```python
from build123d import *

# Parameters (mm, degrees)
F0_R           = 50.8
F1_DEPTH       = 38.1
F3_D           = 6.35
F4_D           = 12.7
F5_D           = 9.525
F5_CBORE_D     = 19.05
F5_CBORE_DEPTH = 6.35
F6_D           = 9.525
F6_CSINK_D     = 19.05
F6_CSINK_ANGLE = 82
F7_D           = 6.35


with BuildPart() as f1:
    # F0 (on Front) → F1 (new body)
    with BuildSketch(Plane.XZ):
        Circle(F0_R)
    extrude(amount=F1_DEPTH)

    # F3 (through all)
    with Locations(Plane(origin=(0, 0, 0), x_dir=(1, 0, 0), z_dir=(0, 1, 0))):
        with Locations((0, -31.75)):
            Hole(F3_D / 2)

    # F4 (through all)
    with Locations(Plane(origin=(0, 0, 0), x_dir=(1, 0, 0), z_dir=(0, 1, 0))):
        with Locations((-28.8894439592, -13.1705173676)):
            Hole(F4_D / 2)

    # F5 (through all)
    with Locations(Plane(origin=(0, 0, 0), x_dir=(1, 0, 0), z_dir=(0, 1, 0))):
        with Locations((28.8894439592, -13.1705173676)):
            CounterBoreHole(F5_D / 2, F5_CBORE_D / 2, F5_CBORE_DEPTH)

    # F6 (through all)
    with Locations(Plane(origin=(0, 0, 0), x_dir=(1, 0, 0), z_dir=(0, 1, 0))):
        with Locations((21.623259188, 23.2485948412)):
            CounterSinkHole(F6_D / 2, F6_CSINK_D / 2, counter_sink_angle=F6_CSINK_ANGLE)

    # F7 (through all)
    with Locations(Plane(origin=(0, 0, 0), x_dir=(1, 0, 0), z_dir=(0, 1, 0))):
        with Locations((-21.623259188, 23.2485948412)):
            Hole(F7_D / 2)


solid = f1.part
```
Geometry check sheet. Reference: the model listing, model coordinates, mm. A direction names the side the tool comes from. Give positions to 0.01 mm unless a question says otherwise; leave off trailing zeros. Order: outer loops, then holes, each group sorted by start corner. A loop starts at its lowest first (then second) coordinate and runs counter-clockwise, first axis right, second up. Notation, with made-up numbers: (-27.5, 75.25) - (24.5, 75.25) arc R30 cw to (24.5, 103.25) - close; hole circle Ø10 at (5.25, -25). An arc over 180 degrees is marked (long way). Answer in a Markdown table with one row per item. Add a question column.
Q1. Cross-section at C-C, the plane y = -13. Count the separate pieces of the cut face and the enclosed holes in it, then the cut area to 3 significant figures.
Q2. Material ranges on probe 1 along X at (y, z) = (-30, 15); probe 2 along Z at (x, y) = (-27, -21); probe 3 along Z at (x, y) = (-32.5, -5.5), recorded low to high. Write a range as from..to.
Q3. Gauge pin test, flat ends, axial feed: pin 1 (8 mm diameter, centred on y = -21.5, z = 15, fed in from +X); pin 2 (11.5 mm diameter, centred on x = -28.89, z = 13.17, fed in from -Y); pin 3 (1 mm diameter, centred on y = -16.5, z = 28.5, fed in from -X); pin 4 (15 mm diameter, centred on x = 28.89, z = 13.17, fed in from +Y). Record the tip position at first contact, or that the pin passes through.
Q4. Mould release check, pull along X, two halves, no side actions. Record for faces 1 (the flat face through (-1, 0, 1)), 2 (the cylindrical face through (-19.1, -19.32, -21.32)), 3 (the cylindrical face through (-11.012, -18.783, -49.592)): pulls with the +X half, pulls with the -X half, needs draft (parallel to the pull), parting line crosses it, or undercut.
Q5. Cross-section at D-D, the plane z = 16. Enter the section's corners in (x, y), then the cut area to 3 significant figures.
Q6. Tool access check on faces 4 (the flat face through (26.6, -6.35, 8.8)), 5 (the cylindrical face through (25.4, -22.02, -20.35)). Record the directions out of +Z, -Z, +X, -X, +Y, -Y that give a thin tool (end or side, any length) a straight path to the whole face; none if there is none.
Q7. Cross-section at B-B, the plane z = 31.75. Enter the section's corners in (x, y) (3 decimals).
Q8. Cross-section at A-A, the plane x = 0. Enter the section's corners in (y, z) (3 decimals).
Check values:
| question | item | result |
|---|---|---|
| 1 | separate pieces | 1 |
| 1 | enclosed holes | 5 |
| 1 | area | 7,770 mm^2 |
| 2 | probe 1 | x = -48.53..-34.97, -22.81..24.49, 33.29..48.53 |
| 2 | probe 2 | z = -43.03..7.11, 19.23..43.03 |
| 2 | probe 3 | z = -39.04..7.95, 18.39..39.04 |
| 3 | pin 1 | stops at x = 49.59 |
| 3 | pin 2 | passes through |
| 3 | pin 3 | stops at x = -42.39 |
| 3 | pin 4 | stops at y = -6.35 |
| 4 | face 1 | needs draft |
| 4 | face 2 | undercut |
| 4 | face 3 | parting line crosses it |
| 5 | outline | (-48.21, -38.1) - (-34.57, -38.1) - (-34.57, 0) - (-48.21, 0) - close; (-23.2, -38.1) - (25.06, -38.1) - (25.06, -6.35) - (19.79, -6.35) - (19.79, 0) - (-23.2, 0) - close; (32.72, -38.1) - (48.21, -38.1) - (48.21, 0) - (37.98, 0) - (37.98, -6.35) - (32.72, -6.35) - close |
| 5 | area | 2,880 mm^2 |
| 6 | face 4 | +Y |
| 6 | face 5 | +Y, -Y |
| 7 | outline | (-39.656, -38.1) - (-3.175, -38.1) - (-3.175, 0) - (-39.656, 0) - close; (3.175, -38.1) - (39.656, -38.1) - (39.656, 0) - (3.175, 0) - close |
| 8 | outline | (-38.1, -50.8) - (0, -50.8) - (0, 28.575) - (-38.1, 28.575) - close; (-38.1, 34.925) - (0, 34.925) - (0, 50.8) - (-38.1, 50.8) - close |
